```python
from build123d import *

# Parameters (mm, degrees)
SKETCH1_R           = 35
SKETCH1_R_2         = 3.5
BOSS_EXTRUDE1_DEPTH = 24
SKETCH3_OUTSIDE_W   = 92.372
SKETCH3_OUTSIDE_H   = 92.372
SKETCH3_OUTSIDE_R   = 32.5
CUT_EXTRUDE1_DEPTH  = 20
CUT_EXTRUDE2_DEPTH  = 20
SKETCH5_R           = 3
CUT_EXTRUDE3_DEPTH  = 56.009090158


with BuildPart() as part:
    # Sketch1 → Boss-Extrude1 (new body)
    with BuildSketch(Plane.XY):
        Circle(SKETCH1_R)
        Circle(SKETCH1_R_2, mode=Mode.SUBTRACT)
    extrude(amount=-BOSS_EXTRUDE1_DEPTH)

    # Sketch3 outside → Cut-Extrude1 (cut)
    with BuildSketch(Plane.XY.offset(-2)):
        Rectangle(SKETCH3_OUTSIDE_W, SKETCH3_OUTSIDE_H)
        Circle(SKETCH3_OUTSIDE_R, mode=Mode.SUBTRACT)
    extrude(amount=-CUT_EXTRUDE1_DEPTH, mode=Mode.SUBTRACT)

    # Sketch4 → Cut-Extrude2 (cut)
    with BuildSketch(Plane.XY.offset(-2)):
        with BuildLine():
            ThreePointArc((-20.684282661, 25.06811622), (-17.923091739, 24.669019428), (-17.449400423, 27.418395738))
            ThreePointArc((-17.449400423, 27.418395738), (-19.1030207, 26.293052317), (-20.684282661, 25.06811622))
        make_face()
        with BuildLine():
            ThreePointArc((-16.508107467, 27.995220804), (-13.84334388, 27.169092131), (-12.945387279, 29.810517409))
            ThreePointArc((-12.945387279, 29.810517409), (-14.754691242, 28.957712036), (-16.508107467, 27.995220804))
        make_face()
        with BuildLine():
            ThreePointArc((-11.925447881, 30.232990141), (-9.422726952, 29.000171617), (-8.122615736, 31.468605206))
            ThreePointArc((-8.122615736, 31.468605206), (-10.043052317, 30.90933678), (-11.925447881, 30.232990141))
        make_face()
        with BuildLine():
            ThreePointArc((-7.049144189, 31.726322923), (-4.770091215, 30.117170631), (-3.099838437, 32.351831504))
            ThreePointArc((-3.099838437, 32.351831504), (-5.084120114, 32.099871069), (-7.049144189, 31.726322923))
        make_face()
        with BuildLine():
            ThreePointArc((-1.999267173, 32.438448341), (-1.394942074, 31.059359006), (0, 30.492584951))
            Line((0, 30.492584951), (0, 32.5))
            ThreePointArc((0, 32.5), (-1.000107224, 32.484608441), (-1.999267173, 32.438448341))
        make_face()
        with BuildLine():
            Line((0, 32.5), (0, 30.492584951))
            ThreePointArc((0, 30.492584951), (1.394942074, 31.059359006), (1.999267173, 32.438448341))
            ThreePointArc((1.999267173, 32.438448341), (1.000107224, 32.484608441), (0, 32.5))
        make_face()
        with BuildLine():
            ThreePointArc((7.049144189, 31.726322923), (5.084120114, 32.099871069), (3.099838437, 32.351831504))
            ThreePointArc((3.099838437, 32.351831504), (4.770091215, 30.117170631), (7.049144189, 31.726322923))
        make_face()
        with BuildLine():
            ThreePointArc((11.925447881, 30.232990141), (10.043052317, 30.90933678), (8.122615736, 31.468605206))
            ThreePointArc((8.122615736, 31.468605206), (9.422726952, 29.000171617), (11.925447881, 30.232990141))
        make_face()
        with BuildLine():
            ThreePointArc((16.508107467, 27.995220804), (14.754691242, 28.957712036), (12.945387279, 29.810517409))
            ThreePointArc((12.945387279, 29.810517409), (13.84334388, 27.169092131), (16.508107467, 27.995220804))
        make_face()
        with BuildLine():
            ThreePointArc((20.684282661, 25.06811622), (19.1030207, 26.293052317), (17.449400423, 27.418395738))
            ThreePointArc((17.449400423, 27.418395738), (17.923091739, 24.669019428), (20.684282661, 25.06811622))
        make_face()
        with BuildLine():
            ThreePointArc((24.351142168, 21.523751418), (22.980970389, 22.980970389), (21.523751418, 24.351142168))
            ThreePointArc((21.523751418, 24.351142168), (21.561513595, 21.561513595), (24.351142168, 21.523751418))
        make_face()
        with BuildLine():
            ThreePointArc((27.418395738, 17.449400423), (26.293052317, 19.1030207), (25.06811622, 20.684282661))
            ThreePointArc((25.06811622, 20.684282661), (24.669019428, 17.923091739), (27.418395738, 17.449400423))
        make_face()
        with BuildLine():
            ThreePointArc((29.810517409, 12.945387279), (28.957712036, 14.754691242), (27.995220804, 16.508107467))
            ThreePointArc((27.995220804, 16.508107468), (27.169092131, 13.84334388), (29.810517409, 12.945387279))
        make_face()
        with BuildLine():
            ThreePointArc((31.468605206, 8.122615736), (30.90933678, 10.043052317), (30.232990141, 11.925447881))
            ThreePointArc((30.232990141, 11.925447881), (29.000171617, 9.422726952), (31.468605206, 8.122615736))
        make_face()
        with BuildLine():
            ThreePointArc((32.351831504, 3.099838437), (32.099871069, 5.084120114), (31.726322923, 7.049144189))
            ThreePointArc((31.726322923, 7.049144189), (30.117170631, 4.770091215), (32.351831504, 3.099838437))
        make_face()
        with BuildLine():
            ThreePointArc((32.5, 0), (32.484608441, 1.000107224), (32.438448341, 1.999267173))
            ThreePointArc((32.438448341, 1.999267173), (30.492584951, 0), (32.438448341, -1.999267173))
            ThreePointArc((32.438448341, -1.999267173), (32.484608441, -1.000107224), (32.5, 0))
        make_face()
        with BuildLine():
            ThreePointArc((31.726322923, -7.049144189), (32.099871069, -5.084120114), (32.351831504, -3.099838437))
            ThreePointArc((32.351831504, -3.099838437), (30.117170631, -4.770091215), (31.726322923, -7.049144189))
        make_face()
        with BuildLine():
            ThreePointArc((30.232990141, -11.925447881), (30.90933678, -10.043052317), (31.468605206, -8.122615736))
            ThreePointArc((31.468605206, -8.122615736), (29.000171617, -9.422726952), (30.232990141, -11.925447881))
        make_face()
        with BuildLine():
            ThreePointArc((27.995220804, -16.508107467), (28.957712036, -14.754691242), (29.810517409, -12.945387279))
            ThreePointArc((29.810517409, -12.945387279), (27.169092131, -13.84334388), (27.995220804, -16.508107467))
        make_face()
        with BuildLine():
            ThreePointArc((25.06811622, -20.684282661), (26.293052317, -19.103020699), (27.418395738, -17.449400423))
            ThreePointArc((27.418395739, -17.449400423), (24.669019428, -17.923091739), (25.06811622, -20.684282661))
        make_face()
        with BuildLine():
            ThreePointArc((21.523751418, -24.351142168), (22.980970389, -22.980970389), (24.351142168, -21.523751418))
            ThreePointArc((24.351142168, -21.523751418), (21.561513595, -21.561513595), (21.523751418, -24.351142168))
        make_face()
        with BuildLine():
            ThreePointArc((17.449400423, -27.418395738), (19.1030207, -26.293052317), (20.684282661, -25.06811622))
            ThreePointArc((20.684282661, -25.06811622), (17.923091739, -24.669019428), (17.449400423, -27.418395738))
        make_face()
        with BuildLine():
            ThreePointArc((12.945387279, -29.810517409), (14.754691242, -28.957712036), (16.508107468, -27.995220804))
            ThreePointArc((16.508107468, -27.995220804), (13.843343881, -27.169092131), (12.945387279, -29.810517409))
        make_face()
        with BuildLine():
            ThreePointArc((8.122615736, -31.468605206), (10.043052317, -30.90933678), (11.925447881, -30.232990141))
            ThreePointArc((11.925447881, -30.232990141), (9.422726952, -29.000171617), (8.122615736, -31.468605206))
        make_face()
        with BuildLine():
            ThreePointArc((3.099838437, -32.351831504), (5.084120114, -32.099871069), (7.049144189, -31.726322923))
            ThreePointArc((7.049144189, -31.726322923), (4.770091215, -30.117170631), (3.099838437, -32.351831504))
        make_face()
        with BuildLine():
            ThreePointArc((1.999267173, -32.438448341), (0, -30.492584951), (-1.999267173, -32.438448341))
            ThreePointArc((-1.999267173, -32.438448341), (0, -32.5), (1.999267173, -32.438448341))
        make_face()
        with BuildLine():
            ThreePointArc((-3.099838437, -32.351831504), (-4.770091215, -30.117170631), (-7.049144189, -31.726322923))
            ThreePointArc((-7.049144189, -31.726322923), (-5.084120114, -32.099871069), (-3.099838437, -32.351831504))
        make_face()
        with BuildLine():
            ThreePointArc((-8.122615736, -31.468605206), (-9.422726952, -29.000171617), (-11.925447881, -30.232990141))
            ThreePointArc((-11.925447881, -30.232990141), (-10.043052317, -30.90933678), (-8.122615736, -31.468605206))
        make_face()
        with BuildLine():
            ThreePointArc((-12.945387279, -29.810517409), (-13.84334388, -27.169092131), (-16.508107467, -27.995220804))
            ThreePointArc((-16.508107467, -27.995220804), (-14.754691242, -28.957712036), (-12.945387279, -29.810517409))
        make_face()
        with BuildLine():
            ThreePointArc((-17.449400423, -27.418395738), (-17.923091739, -24.669019428), (-20.684282661, -25.06811622))
            ThreePointArc((-20.684282661, -25.06811622), (-19.103020699, -26.293052317), (-17.449400423, -27.418395738))
        make_face()
        with BuildLine():
            ThreePointArc((-21.523751418, -24.351142168), (-21.561513595, -21.561513595), (-24.351142168, -21.523751418))
            ThreePointArc((-24.351142168, -21.523751418), (-22.980970389, -22.980970389), (-21.523751418, -24.351142168))
        make_face()
        with BuildLine():
            ThreePointArc((-25.06811622, -20.684282661), (-24.669019428, -17.923091739), (-27.418395738, -17.449400423))
            ThreePointArc((-27.418395738, -17.449400423), (-26.293052317, -19.1030207), (-25.06811622, -20.684282661))
        make_face()
        with BuildLine():
            ThreePointArc((-27.995220804, -16.508107468), (-27.169092131, -13.84334388), (-29.810517409, -12.945387279))
            ThreePointArc((-29.810517409, -12.945387279), (-28.957712036, -14.754691242), (-27.995220804, -16.508107468))
        make_face()
        with BuildLine():
            ThreePointArc((-30.232990141, -11.925447881), (-29.000171617, -9.422726952), (-31.468605206, -8.122615736))
            ThreePointArc((-31.468605206, -8.122615736), (-30.90933678, -10.043052317), (-30.232990141, -11.925447881))
        make_face()
        with BuildLine():
            ThreePointArc((-31.726322923, -7.049144189), (-30.117170631, -4.770091215), (-32.351831504, -3.099838437))
            ThreePointArc((-32.351831504, -3.099838437), (-32.099871069, -5.084120114), (-31.726322923, -7.049144189))
        make_face()
        with BuildLine():
            ThreePointArc((-32.438448341, -1.999267173), (-30.492584951, 0), (-32.438448341, 1.999267173))
            ThreePointArc((-32.438448341, 1.999267173), (-32.5, 0), (-32.438448341, -1.999267173))
        make_face()
        with BuildLine():
            ThreePointArc((-32.351831504, 3.099838437), (-30.117170631, 4.770091215), (-31.726322923, 7.049144189))
            ThreePointArc((-31.726322923, 7.049144189), (-32.099871069, 5.084120114), (-32.351831504, 3.099838437))
        make_face()
        with BuildLine():
            ThreePointArc((-31.468605206, 8.122615736), (-29.000171617, 9.422726952), (-30.232990141, 11.925447881))
            ThreePointArc((-30.232990141, 11.925447881), (-30.90933678, 10.043052317), (-31.468605206, 8.122615736))
        make_face()
        with BuildLine():
            ThreePointArc((-29.810517409, 12.945387279), (-27.169092131, 13.84334388), (-27.995220804, 16.508107467))
            ThreePointArc((-27.995220804, 16.508107467), (-28.957712036, 14.754691242), (-29.810517409, 12.945387279))
        make_face()
        with BuildLine():
            ThreePointArc((-27.418395738, 17.449400423), (-24.669019428, 17.923091739), (-25.06811622, 20.684282661))
            ThreePointArc((-25.06811622, 20.684282661), (-26.293052317, 19.103020699), (-27.418395738, 17.449400423))
        make_face()
        with BuildLine():
            ThreePointArc((-24.351142168, 21.523751418), (-21.561513595, 21.561513595), (-21.523751418, 24.351142168))
            ThreePointArc((-21.523751418, 24.351142168), (-22.980970389, 22.980970389), (-24.351142168, 21.523751418))
        make_face()
    extrude(amount=-CUT_EXTRUDE2_DEPTH, mode=Mode.SUBTRACT)

    # Sketch5 → Cut-Extrude3 (cut, through all)
    with BuildSketch(Plane(origin=(0, 0, 0), x_dir=(1, 0, 0), z_dir=(0, 1, 0))):
        with Locations(Location((0, 12.279237026, 0), (0, 0, 90))):
            Circle(SKETCH5_R)
    extrude(amount=CUT_EXTRUDE3_DEPTH, mode=Mode.SUBTRACT)


solid = part.part
```
Geometry check sheet. Reference: the model listing, model coordinates, mm. A direction names the side the tool comes from. Coordinates: 2 decimals unless noted, no trailing zeros. Order: outer loops, then holes, each group sorted by start corner. A loop starts at its lowest first (then second) coordinate and runs counter-clockwise, first axis right, second up.
Item 1: Tool access check on faces 1 (the cylindrical face through (1.15, 16.91, -15.05)), 2 (the cylindrical face through (-27.189, 13.805, -11.86)), 3 (the cylindrical face through (0.043, -30.493, -11.86)), 4 (the cylindrical face through (-0.759, -3.417, -11.832)). Record the directions out of +Z, -Z, +X, -X, +Y, -Y that give a thin tool (end or side, any length) a straight path to the whole face; none if there is none.
Item 2: Section check C-C (y = -15). Enter the section's corners in (x, z).
Item 3: Section check B-B (y = 19). Enter the section's corners in (x, z), plus the area to 3 significant figures.
Item 4: Depth check by flat-ended pin: pin 1 (10 mm diameter, centred on x = 8.5, z = -14, fed in from +Y); pin 2 (5 mm diameter, centred on y = 23, z = -9.5, fed in from +X); pin 3 (10 mm diameter, centred on x = 3.5, z = -8.5, fed in from -Y). Enter the tip coordinate at first touch or a pass-through.
Item 5: Section check A-A (y = 0). Enter the section's corners in (x, z), plus the area to 3 significant figures.
Item 6: Mould release check, pull along X, two halves, no side actions. Record for faces 5 (the cylindrical face through (17.958, -24.644, -11.86)), 6 (the cylindrical face through (-30.493, -0.043, -11.86)): released by +X, released by -X, zero draft, split by the parting line, or undercut.
Item 7: Scan lines: line 1 along X through (y, z) = (31, -8.5); line 2 along X through (y, z) = (31, -12); line 3 along X through (y, z) = (10, -4.5). Record each from-to range of solid material in increasing order.
Check sheet entries:
1. face 1: +Y
1. face 2: none
1. face 3: -Y
1. face 4: +Z, -Z
2. outline: (-31.62, -24) - (31.62, -24) - (31.62, -22) - (26.97, -22) - (26.97, -2) - (31.62, -2) - (31.62, 0) - (-31.62, 0) - (-31.62, -2) - (-26.97, -2) - (-26.97, -22) - (-31.62, -22) - close
3. outline: (-29.39, -24) - (29.39, -24) - (29.39, -22) - (24.29, -22) - (24.29, -2) - (29.39, -2) - (29.39, 0) - (-29.39, 0) - (-29.39, -2) - (-24.29, -2) - (-24.29, -22) - (-29.39, -22) - close; hole circle Ø6 at (0, -12.28)
3. area: 1,180 mm2
4. pin 1: stops at y = 31.73
4. pin 2: stops at x = 25.07
4. pin 3: stops at y = -32.44
5. outline: (-35, -24) - (-3.5, -24) - (-3.5, 0) - (-35, 0) - (-35, -2) - (-30.49, -2) - (-30.49, -22) - (-35, -22) - close; (3.5, -24) - (35, -24) - (35, -22) - (30.49, -22) - (30.49, -2) - (35, -2) - (35, 0) - (3.5, 0) - close
5. area: 1,330 mm2
6. face 5: undercut
6. face 6: released by -X
7. line 1: x = -8.04 to -6.76, -3.41 to -1.33, 1.33 to 3.41, 6.76 to 8.04
7. line 2: x = -8.04 to -6.76, -3.41 to -2.99, 2.99 to 3.41, 6.76 to 8.04
7. line 3: x = -28.9 to 28.9
